The model under review builds one solid part; all positions refer to its coordinate system, in mm. A direction names the side the tool comes from. Coordinates: 2 decimals unless noted, no trailing zeros. Order: outer loops, then holes, each group sorted by start corner. A loop starts at its lowest first (then second) coordinate and runs counter-clockwise, first axis right, second up. Notation, with made-up numbers: (72.5, 8.25) -> (124.5, 8.25) arc R25 ccw to (124.5, 40.25) -> close; hole circle Ø9 at (25.25, 14.5). An arc over 180 degrees is marked (long way). Use one line per item in the form item = value. Start each with the question number.
(1) Take a section at B-B (x = -63.5). State the section outline as (y, z) points (3 decimals).
(2) Insertion check: pin 1 Ø5 at (x, y) = (-46.5, -33.5) entering from +Z. The pin has a flat end and moves straight along its axis. Give the tip position at first contact, or say it passes through.
(3) Wall thickness on line 1 along X through (y, z) = (69.5, 6); line 2 along Z through (x, y) = (-26.5, -53.5); line 3 along X through (y, z) = (14.5, 10): over which ranges is each line inside the solid? List them lowest first.
(4) Take a section at C-C (y = -29.5). State the section outline as (x, z) points, then the cut area to 3 significant figures.
(5) Take a section at A-A (z = 2). State the section outline as (x, y) points.
(6) For faces 1 (the flat face through (76.2, -1, 0)), 2 (the flat face through (-57, 57, 0)), list the 3-axis set-ups (+Z, -Z, +X, -X, +Y, -Y) from which the entire face can be reached by the end or side of a thin tool; tool diameter is ignored.
(7) Mouldability with a two-part tool opening along Y and no side actions: class faces 3 (the flat face through (-44.45, 57, 3)), 4 (the flat face through (-69.85, 57, 3)), 5 (the flat face through (-1, 76.2, 0)), 6 (the flat face through (-1, -76.2, 0)) as +Y half, -Y half, draft (parallel to the pull), parting line (faces both ways), or undercut.
(8) Take a section at D-D (z = 32). State the section outline as (x, y) points (1 decimal).
```python
from build123d import *

# Parameters (mm, degrees)
F0_W     = 152.4
F0_H     = 152.4
F1_DEPTH = 6.35
F2_W     = 25.4
F2_H     = 25.4
F3_DEPTH = 6.35
F5_W     = 7.9375
F5_H     = 28.575


with BuildPart() as f1:
    # F0 (on Top) → F1 (new body, symmetric)
    with BuildSketch(Plane.XY):
        Rectangle(F0_W, F0_H)
    extrude(amount=F1_DEPTH, both=True)

    # F2 (on face) → F3 (cut)
    with BuildSketch(Plane.XY.offset(6.35)):
        with Locations((-57.15, 57.15)):
            Rectangle(F2_W, F2_H)
    extrude(amount=-F3_DEPTH, mode=Mode.SUBTRACT)

    # F5 (on offset) → F6 (revolve)
    with BuildSketch(Plane.YZ.offset(-63.5)):
        with Locations((15.678355, 20.6375)):
            Rectangle(F5_W, F5_H)
    revolve(axis=Axis((-63.5, 11.709605, 20.6375), (0, 0, 1)))


solid = f1.part
```
Findings:
q1.outline = (-76.2, -6.35) -> (76.2, -6.35) -> (76.2, 6.35) -> (69.85, 6.35) -> (69.85, 0) -> (44.45, 0) -> (44.45, 6.35) -> (19.647, 6.35) -> (19.647, 34.925) -> (3.772, 34.925) -> (3.772, 6.35) -> (-76.2, 6.35) -> close
q2.pin_1 = 6.35
q3.line_1 = -76.2 to -69.85, -44.45 to 76.2
q3.line_2 = -6.35 to 6.35
q3.line_3 = -70.93 to -56.07
q4.outline = (-76.2, -6.35) -> (76.2, -6.35) -> (76.2, 6.35) -> (-76.2, 6.35) -> close
q4.area = 1,940 mm²
q5.outline = (-76.2, -76.2) -> (76.2, -76.2) -> (76.2, 76.2) -> (-76.2, 76.2) -> close; hole (-69.85, 44.45) -> (-44.45, 44.45) -> (-44.45, 69.85) -> (-69.85, 69.85) -> close
q6.face_1 = +Z, -Z, +X, +Y, -Y
q6.face_2 = +Z
q7.face_3 = undercut
q7.face_4 = undercut
q7.face_5 = +Y half
q7.face_6 = -Y half
q8.outline = circle Ø15.9 at (-63.5, 11.7)
